Design review of the part built by this model. Coordinates are the model's own, in mm. Give positions to 0.01 mm unless a question says otherwise; leave off trailing zeros. Loops run counter-clockwise (first coordinate to the right, second up) from the corner with the lowest first, then second, coordinate; pieces in that order, holes last.
from build123d import *

# Parameters (mm, degrees)
SKETCH1_W                  = 12.7
SKETCH1_H                  = 76.2
EXTRUDE1_DEPTH             = 6.35
F_10_32_TAPPED_HOLE1_D     = 4.0386
F_10_32_TAPPED_HOLE1_DEPTH = 13.716
F_10_32_TAPPED_HOLE1_TIP   = 1.213317848
FILLET1_R                  = 1.5875


with BuildPart() as part:
    # Sketch1 → Extrude1 (new body)
    with BuildSketch(Plane.XY):
        with Locations((0, 38.1)):
            Rectangle(SKETCH1_W, SKETCH1_H)
    extrude(amount=-EXTRUDE1_DEPTH)

    # #10-32 Tapped Hole1
    with Locations(Plane.XY):
        with Locations((0, 57.15), (0, 19.05)):
            Hole(F_10_32_TAPPED_HOLE1_D / 2, depth=F_10_32_TAPPED_HOLE1_DEPTH)
            with Locations((0, 0, -(F_10_32_TAPPED_HOLE1_DEPTH + F_10_32_TAPPED_HOLE1_TIP / 2))):  # 118° drill point
                Cone(0, F_10_32_TAPPED_HOLE1_D / 2, F_10_32_TAPPED_HOLE1_TIP, mode=Mode.SUBTRACT)

    # Fillet1
    fillet1_edges = [part.edges().sort_by_distance(p)[0] for p in [
        (-6.35, 76.2, -3.175),
        (6.35, 76.2, -3.175),
        (6.35, 0, -3.175),
        (-6.35, 0, -3.175),
    ]]
    fillet(fillet1_edges, radius=FILLET1_R)


solid = part.part
Q1. Take a section at C-C (z = -2.25). Give the number of separate pieces and of enclosed holes in the cut face, plus the area to 3 significant figures.
Results:
separate pieces: 1
enclosed holes: 2
area: 940 mm2
Q2. Take a section at B-B (y = 19.05). Give the boundary of the cut face in (x, z).
Results:
outline: (-6.35, -6.35) - (-2.02, -6.35) - (-2.02, 0) - (-6.35, 0) - close; (2.02, -6.35) - (6.35, -6.35) - (6.35, 0) - (2.02, 0) - close
Q3. Wall thickness on line 1 (Y direction, x = 0, z = -3.25); line 2 (Y direction, x = -1, z = -3.5); line 3 (X direction, y = 58, z = -2.25): over which ranges is each line inside the solid? List them lowest first.
Results:
line 1: y = 0 to 17.03, 21.07 to 55.13, 59.17 to 76.2
line 2: y = 0 to 17.3, 20.8 to 55.4, 58.9 to 76.2
line 3: x = -6.35 to -1.83, 1.83 to 6.35
Q4. Take a section at A-A (x = 0). Give the boundary of the cut face in (y, z).
Results:
outline: (0, -6.35) - (17.03, -6.35) - (17.03, 0) - (0, 0) - close; (21.07, -6.35) - (55.13, -6.35) - (55.13, 0) - (21.07, 0) - close; (59.17, -6.35) - (76.2, -6.35) - (76.2, 0) - (59.17, 0) - close
Q5. Draft analysis for pull direction Y (two halves, no side actions). For faces 1 (the face through (0, 0, -3)), 2 (the face through (-1.09, 58.85, -3.22)), 3 (the face through (-5.9, 75.72, -3.22)), 4 (the face through (0.44, 17.08, -3.22)), state which applies: pulls with the +Y half, pulls with the -Y half, needs draft (parallel to the pull), parting line crosses it, or undercut.
Results:
face 1: pulls with the -Y half
face 2: undercut
face 3: pulls with the +Y half
face 4: undercut
